Source: CAD feature listing. Evaluate the final solid. Frame: model axes, mm. A direction names the side the tool comes from. Round coordinates to 2 decimals unless told otherwise and drop trailing zeros. Write each loop counter-clockwise with the first axis right and the second up, starting at its lowest first coordinate (ties: lowest second). Pieces come first, ordered by that corner, then holes. Notation, with made-up numbers: (-16.75, 33.25) -> (11.25, 33.25) arc R17 ccw to (11.25, 55.25) -> close; hole circle Ø4 at (11.5, -33). An arc over 180 degrees is marked (long way). Put each result on its own line as item: value.
```python
from build123d import *

# Parameters (mm, degrees)
BOSS_EXTRUDE1_DEPTH = 38.1
FILLET1_R           = 2.54
SKETCH2_R           = 2.54
CUT_EXTRUDE1_DEPTH  = 329.417801017


with BuildPart() as part:
    # Sketch1 → Boss-Extrude1 (new body)
    with BuildSketch(Plane.XY):
        Polygon((-50.8, -1.905), (50.8, -1.905), (148.59, -90.805), (148.59, -116.205), (152.4, -116.205), (152.4, -90.805), (50.8, 1.905), (-50.8, 1.905), (-152.4, -90.805), (-152.4, -116.205), (-148.59, -116.205), (-148.59, -90.805), align=None)
    extrude(amount=-BOSS_EXTRUDE1_DEPTH)

    # Fillet1
    fillet1_edges = [part.edges().sort_by_distance(p)[0] for p in [
        (152.4, -90.805, -19.05),
        (148.59, -90.805, -19.05),
        (50.8, -1.905, -19.05),
        (-50.8, -1.905, -19.05),
        (-148.59, -90.805, -19.05),
        (-152.4, -90.805, -19.05),
        (-50.8, 1.905, -19.05),
        (50.8, 1.905, -19.05),
    ]]
    fillet(fillet1_edges, radius=FILLET1_R)

    # Sketch2 → Cut-Extrude1 (cut, through all)
    with BuildSketch(Plane(origin=(152.4, 0, 0), x_dir=(0, 0, -1), z_dir=(1, 0, 0))):
        with Locations((19.05, -104.065395562)):
            Circle(SKETCH2_R)
    extrude(amount=-CUT_EXTRUDE1_DEPTH, mode=Mode.SUBTRACT)


solid = part.part
```
Q1. Draft query along Z for faces 1 (the flat face through (-1, 0, -38.1)), 2 (the flat face through (98.969, -45.695, -18.783)), 3 (the cylindrical face through (150.522, -101.547, -18.719)). Return one class per face: +Z half, -Z half, draft (parallel to the pull), parting line (faces both ways), or undercut.
Ans:
face 1: -Z half
face 2: draft
face 3: undercut
Q2. Cut plane C-C on x = -121.5. Output: boundary loops of the cut face in (y, z).
Ans:
outline: (-66.18, -38.1) -> (-62.61, -38.1) -> (-62.61, 0) -> (-66.18, 0) -> close
Q3. Pin query (flat end, axial travel): pin 1 (6 mm diameter, centred on x = -107, z = -31.5, fed in from +Y); pin 2 (12 mm diameter, centred on x = 72, z = -8.5, fed in from +Y) (3 decimals); pin 3 (11.5 mm diameter, centred on x = -2, z = -15, fed in from -Y) (3 decimals). Return the tip coordinate at first contact, or that it passes through.
Ans:
pin 1: stops at y = -46.64
pin 2: stops at y = -11.965
pin 3: stops at y = -1.905
Q4. Cut plane D-D on x = 103. Output: boundary loops of the cut face in (y, z), and give its area (3 significant figures).
Ans:
outline: (-49.36, -38.1) -> (-45.73, -38.1) -> (-45.73, 0) -> (-49.36, 0) -> close
area: 138 mm^2
Q5. Reachability of faces 4 (the flat face through (148.59, -101, -19)), 5 (the flat face through (-1, 0, 0)) from +Z, -Z, +X, -X, +Y, -Y: full face, straight path, thin tool, end or side. Return the list, or none.
Ans:
face 4: +Z, -Z, -Y
face 5: +Z, +X, -X, +Y, -Y
Q6. Material intervals for line 1 (X direction, y = -93, z = -15); line 2 (Y direction, x = -150, z = -19) (3 decimals); line 3 (X direction, y = -39, z = -9), sorted ascending. Write a range as [from, to].
Ans:
line 1: x = [-152.4, -148.59], [148.59, 152.4]
line 2: y = [-116.205, -106.605], [-101.526, -88.615]
line 3: x = [-95.63, -91.6], [91.6, 95.63]
Q7. Cut plane B-B on z = -12. Output: boundary loops of the cut face in (x, y) (3 decimals).
Ans:
outline: (-152.4, -116.205) -> (-148.59, -116.205) -> (-148.59, -91.929) arc R2.54 cw to (-147.759, -90.049) -> (-51.527, -2.566) arc R2.54 cw to (-49.818, -1.905) -> (49.818, -1.905) arc R2.54 cw to (51.527, -2.566) -> (147.759, -90.049) arc R2.54 cw to (148.59, -91.929) -> (148.59, -116.205) -> (152.4, -116.205) -> (152.4, -91.926) arc R2.54 ccw to (151.572, -90.05) -> (51.527, 1.241) arc R2.54 ccw to (49.815, 1.905) -> (-49.815, 1.905) arc R2.54 ccw to (-51.527, 1.241) -> (-151.572, -90.05) arc R2.54 ccw to (-152.4, -91.926) -> close
Q8. Cut plane A-A on y = -58.5. Output: boundary loops of the cut face in (x, z).
Ans:
outline: (-117, -38.1) -> (-113.05, -38.1) -> (-113.05, 0) -> (-117, 0) -> close; (113.05, -38.1) -> (117, -38.1) -> (117, 0) -> (113.05, 0) -> close
